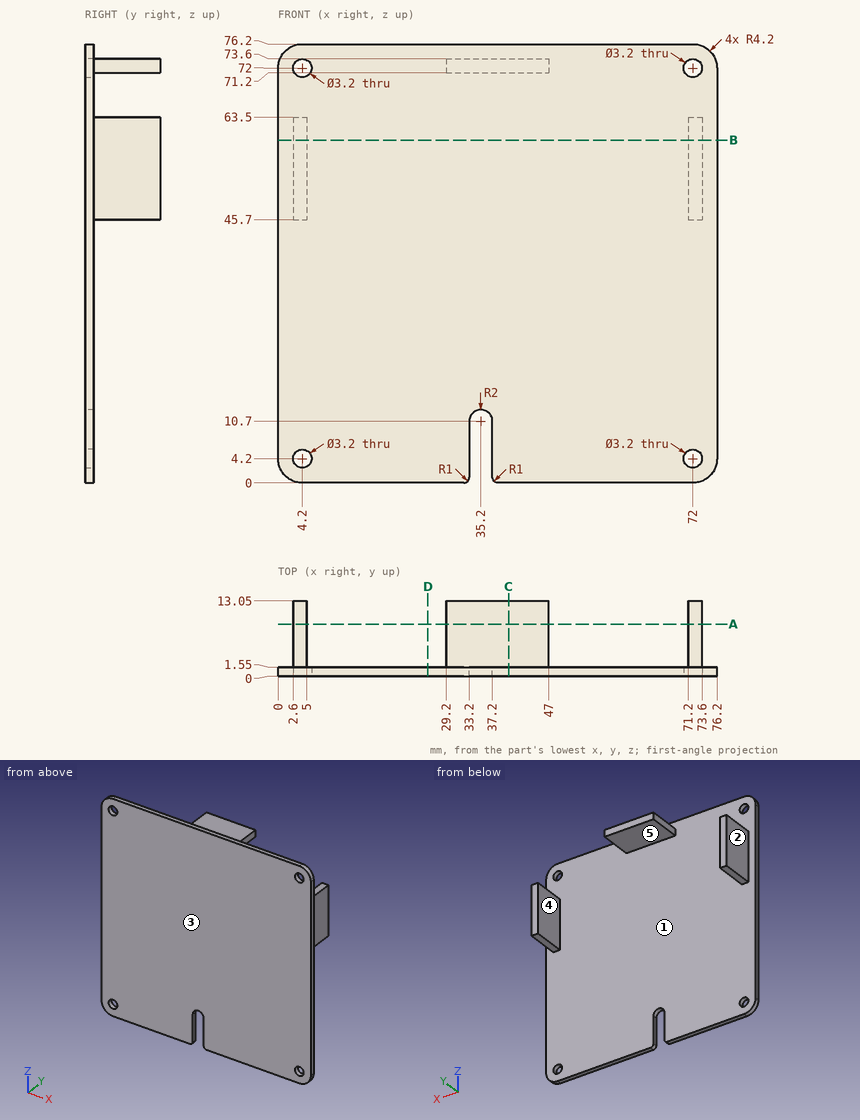
Design review of the part shown in the three views and the two pictorial views. Dimensions are in mm from the part's minimum x, y and z. A direction names the side the tool comes from. Coordinates: 2 decimals unless noted, no trailing zeros. Order: outer loops, then holes, each group sorted by start corner. A loop starts at its lowest first (then second) coordinate and runs counter-clockwise, first axis right, second up. Notation, with made-up numbers: (88.25, -20) -> (123.25, -20) arc R21 ccw to (123.25, -3) -> close; hole circle Ø6 at (7, 2.25). An arc over 180 degrees is marked (long way). Use one line per item in the form item = value. Start each with the question number.
(1) Insertion check: pin 1 (0.7 mm diameter, centred on x = 72.5, y = 4.5, fed in from +Z); pin 2 (6 mm diameter, centred on x = 41, y = 9, fed in from +Z); pin 3 (8 mm diameter, centred on x = 30, z = 60.5, fed in from -Y); pin 4 (1.2 mm diameter, centred on x = 72.5, y = 5.5, fed in from -Z). Each pin has a flat end and moves straight along its axis. Give the tip position at first contact, or say it passes through.
(2) For the marked faces 4 and 5, list the 3-axis set-ups (+Z, -Z, +X, -X, +Y, -Y) from which the entire face can be reached by the end or side of a thin tool; tool diameter is ignored.
(3) For probe 1 along Z at (x, y) = (72, 0.55); probe 2 along X at (y, z) = (12.5, 55), list the stretches that pass through material, from the lowest coordinate up.
(4) Add section D-D on x = 26. State the section outline as (y, z) points, plus the area to 3 significant figures.
(5) Add section B-B on z = 59.5. State the section outline as (x, y) points, plus the area to 3 significant figures.
(6) The part is to be moulded in two halves that separate along X. For the marked faces 1, 2 and 3, say which applies: +X half, -X half, draft (parallel to the pull), parting line (faces both ways), or undercut.
(7) Add section C-C on x = 40. State the section outline as (y, z) points, plus the area to 3 significant figures.
(8) Add section A-A on y = 9. State the section outline as (x, z) points.
Answer block:
q1.pin_1 = 63.5
q1.pin_2 = 73.6
q1.pin_3 = 0
q1.pin_4 = 45.7
q2.face_4 = +Z, -Z, +Y
q2.face_5 = -Z, +X, -X, +Y
q3.probe_1 = 0 to 2.6, 5.8 to 70.4, 73.6 to 76.2
q3.probe_2 = 2.6 to 5, 71.2 to 73.6
q4.outline = (0, 0) -> (1.55, 0) -> (1.55, 76.2) -> (0, 76.2) -> close
q4.area = 118 mm²
q5.outline = (0, 0) -> (76.2, 0) -> (76.2, 1.55) -> (73.6, 1.55) -> (73.6, 13.05) -> (71.2, 13.05) -> (71.2, 1.55) -> (5, 1.55) -> (5, 13.05) -> (2.6, 13.05) -> (2.6, 1.55) -> (0, 1.55) -> close
q5.area = 173 mm²
q6.face_1 = undercut
q6.face_2 = -X half
q6.face_3 = draft
q7.outline = (0, 0) -> (1.55, 0) -> (1.55, 71.2) -> (13.05, 71.2) -> (13.05, 73.6) -> (1.55, 73.6) -> (1.55, 76.2) -> (0, 76.2) -> close
q7.area = 146 mm²
q8.outline = (2.6, 45.7) -> (5, 45.7) -> (5, 63.5) -> (2.6, 63.5) -> close; (29.2, 71.2) -> (47, 71.2) -> (47, 73.6) -> (29.2, 73.6) -> close; (71.2, 45.7) -> (73.6, 45.7) -> (73.6, 63.5) -> (71.2, 63.5) -> close
